```python
from build123d import *

# Parameters (mm, degrees)
SKETCH2_W           = 69.98716
SKETCH2_H           = 21.7678
BOSS_EXTRUDE1_DEPTH = 1.016
SKETCH3_W           = 67.6656
SKETCH3_H           = 19.4818
BOSS_EXTRUDE2_DEPTH = 1.524
FILLET1_R           = 1.27


with BuildPart() as part:
    # Sketch2 → Boss-Extrude1 (new body)
    with BuildSketch(Plane(origin=(0, 0, 0), x_dir=(1, 0, 0), z_dir=(0, 1, 0))):
        with Locations((34.99358, 10.8839)):
            Rectangle(SKETCH2_W, SKETCH2_H)
    extrude(amount=BOSS_EXTRUDE1_DEPTH)

    # Sketch3 → Boss-Extrude2 (add)
    with BuildSketch(Plane(origin=(0, 1.016, 0), x_dir=(1, 0, 0), z_dir=(0, 1, 0))):
        with Locations((34.9758, 10.8839)):
            Rectangle(SKETCH3_W, SKETCH3_H)
    extrude(amount=BOSS_EXTRUDE2_DEPTH)

    # Fillet1
    fillet1_edges = [part.edges().sort_by_distance(p)[0] for p in [
        (1.143, 1.778, -20.6248),
        (1.143, 1.778, -1.143),
        (68.8086, 1.778, -1.143),
        (68.8086, 1.778, -20.6248),
        (0, 0.508, -21.7678),
        (69.98716, 0.508, -21.7678),
        (69.98716, 0.508, 0),
        (0, 0.508, 0),
    ]]
    fillet(fillet1_edges, radius=FILLET1_R)


solid = part.part
```
Verification items for the finished model (mm, model axes). A direction names the side the tool comes from. Coordinates: 2 decimals unless noted, no trailing zeros. Loops run counter-clockwise (first coordinate to the right, second up) from the corner with the lowest first, then second, coordinate; pieces in that order, holes last. Notation, with made-up numbers: (47.5, -7.75) - (81.5, -7.75) arc R22 ccw to (81.5, -1.75) - close; hole circle Ø5 at (3, 55.5). An arc over 180 degrees is marked (long way). Answer as a JSON object with one key per item and string values.
(1) Cross-section at B-B, the plane x = 64. Record the boundary of the cut face in (y, z), then the cut area to 3 significant figures.
Response:
{"outline": "(0, -21.77) - (1.02, -21.77) - (1.02, -20.62) - (2.54, -20.62) - (2.54, -1.14) - (1.02, -1.14) - (1.02, 0) - (0, 0) - close", "area": "51.8 mm²"}
(2) Go/stop test with flat-tipped pins: pin 1 Ø0.5 at (x, y) = (44, 1.5) entering from +Z; pin 2 Ø0.8 at (y, z) = (2, -8) entering from +X; pin 3 Ø0.8 at (y, z) = (1.5, -11) entering from -X. Record where each tip stops, or that it passes through.
Response:
{"pin 1": "stops at z = -1.14", "pin 2": "stops at x = 68.81", "pin 3": "stops at x = 1.14"}
(3) Cross-section at A-A, the plane y = 1.7. Record the boundary of the cut face in (x, z).
Response:
{"outline": "(1.14, -19.35) arc R1.27 ccw to (2.41, -20.62) - (67.54, -20.62) arc R1.27 ccw to (68.81, -19.35) - (68.81, -2.41) arc R1.27 ccw to (67.54, -1.14) - (2.41, -1.14) arc R1.27 ccw to (1.14, -2.41) - close"}
(4) Access from +Z, -Z, +X, -X, +Y, -Y to the whole of each face (thin tool, end or side, straight path). Record for faces 1 (the flat face through (35, 2, -1.143)), 2 (the cylindrical face through (68.43, 1.79, -1.51)), 3 (the flat face through (68.809, 2, -11)), 4 (the cylindrical face through (1.52, 1.79, -1.51)).
Response:
{"face 1": "+Z, +X, -X, +Y", "face 2": "+Z, +X, +Y", "face 3": "+Z, -Z, +X, +Y", "face 4": "+Z, -X, +Y"}
(5) Scan lines: line 1 along Z through (x, y) = (57, 1.05); line 2 along X through (y, z) = (1.6, -5.5); line 3 along X through (y, z) = (2.05, -1.25). Record each from-to range of solid material in increasing order.
Response:
{"line 1": "z = -20.62 to -1.14", "line 2": "x = 1.14 to 68.81", "line 3": "x = 1.9 to 68.05"}
